```python
from build123d import *

# Parameters (mm, degrees)
SKETCH1_R               = 1.5
BOSS_EXTRUDE1_DEPTH     = 3.18
SKETCH1_6_R             = 1.5
BOSS_EXTRUDE2_DEPTH     = 1.59
CUT_EXTRUDE1_DEPTH      = 183.307082693
CUT_EXTRUDE1_DEPTH_BACK = 183.307082693
SKETCH2_R               = 1.725


with BuildPart() as part:
    # Sketch1 → Boss-Extrude1 (new body)
    with BuildSketch(Plane.XY):
        Polygon((46.2, 0), (0, 0), (0, -60), (46.2, -60), (46.2, -100), (106.2, -100), (106.2, -60), (152.4, -60), (152.4, 0), (106.2, 0), (106.2, 40), (46.2, 40), align=None)
        with Locations(Location((7.62, -55, 0), (0, 0, 180))):
            Circle(SKETCH1_R, mode=Mode.SUBTRACT)
        with Locations(Location((22.86, -55, 0), (0, 0, 180))):
            Circle(SKETCH1_R, mode=Mode.SUBTRACT)
        with Locations(Location((7.62, -45, 0), (0, 0, 180))):
            Circle(SKETCH1_R, mode=Mode.SUBTRACT)
        with Locations(Location((7.62, -35, 0), (0, 0, 180))):
            Circle(SKETCH1_R, mode=Mode.SUBTRACT)
        with Locations(Location((38.1, -55, 0), (0, 0, 180))):
            Circle(SKETCH1_R, mode=Mode.SUBTRACT)
        with Locations(Location((53.34, -55, 0), (0, 0, 180))):
            Circle(SKETCH1_R, mode=Mode.SUBTRACT)
        with Locations(Location((68.58, -55, 0), (0, 0, 180))):
            Circle(SKETCH1_R, mode=Mode.SUBTRACT)
        with Locations(Location((83.82, -55, 0), (0, 0, 180))):
            Circle(SKETCH1_R, mode=Mode.SUBTRACT)
        with Locations(Location((99.06, -55, 0), (0, 0, 180))):
            Circle(SKETCH1_R, mode=Mode.SUBTRACT)
        with Locations(Location((114.3, -55, 0), (0, 0, 180))):
            Circle(SKETCH1_R, mode=Mode.SUBTRACT)
        with Locations(Location((129.54, -55, 0), (0, 0, 180))):
            Circle(SKETCH1_R, mode=Mode.SUBTRACT)
        with Locations(Location((144.78, -55, 0), (0, 0, 180))):
            Circle(SKETCH1_R, mode=Mode.SUBTRACT)
        with Locations(Location((144.78, -45, 0), (0, 0, 180))):
            Circle(SKETCH1_R, mode=Mode.SUBTRACT)
        with Locations(Location((144.78, -35, 0), (0, 0, 180))):
            Circle(SKETCH1_R, mode=Mode.SUBTRACT)
        with Locations(Location((7.62, -25, 0), (0, 0, 180))):
            Circle(SKETCH1_R, mode=Mode.SUBTRACT)
        with Locations(Location((7.62, -15, 0), (0, 0, 180))):
            Circle(SKETCH1_R, mode=Mode.SUBTRACT)
        with Locations(Location((7.62, -5, 0), (0, 0, 180))):
            Circle(SKETCH1_R, mode=Mode.SUBTRACT)
        with Locations(Location((22.86, -5, 0), (0, 0, 180))):
            Circle(SKETCH1_R, mode=Mode.SUBTRACT)
        with Locations(Location((38.1, -5, 0), (0, 0, 180))):
            Circle(SKETCH1_R, mode=Mode.SUBTRACT)
        with Locations(Location((53.34, -5, 0), (0, 0, 180))):
            Circle(SKETCH1_R, mode=Mode.SUBTRACT)
        with Locations(Location((99.06, -5, 0), (0, 0, 180))):
            Circle(SKETCH1_R, mode=Mode.SUBTRACT)
        with Locations(Location((144.78, -25, 0), (0, 0, 180))):
            Circle(SKETCH1_R, mode=Mode.SUBTRACT)
        with Locations(Location((144.78, -15, 0), (0, 0, 180))):
            Circle(SKETCH1_R, mode=Mode.SUBTRACT)
        with Locations(Location((114.3, -5, 0), (0, 0, 180))):
            Circle(SKETCH1_R, mode=Mode.SUBTRACT)
        with Locations(Location((129.54, -5, 0), (0, 0, 180))):
            Circle(SKETCH1_R, mode=Mode.SUBTRACT)
        with Locations(Location((144.78, -5, 0), (0, 0, 180))):
            Circle(SKETCH1_R, mode=Mode.SUBTRACT)
        with Locations(Location((99.06, 35, 0), (0, 0, 180))):
            Circle(SKETCH1_R, mode=Mode.SUBTRACT)
        with Locations(Location((53.34, 8.333333333, 0), (0, 0, 180))):
            Circle(SKETCH1_R, mode=Mode.SUBTRACT)
        with Locations(Location((53.34, 21.666666667, 0), (0, 0, 180))):
            Circle(SKETCH1_R, mode=Mode.SUBTRACT)
        with Locations(Location((53.34, 35, 0), (0, 0, 180))):
            Circle(SKETCH1_R, mode=Mode.SUBTRACT)
        with Locations(Location((68.58, 35, 0), (0, 0, 180))):
            Circle(SKETCH1_R, mode=Mode.SUBTRACT)
        with Locations(Location((99.06, 8.333333333, 0), (0, 0, 180))):
            Circle(SKETCH1_R, mode=Mode.SUBTRACT)
        with Locations(Location((99.06, 21.666666667, 0), (0, 0, 180))):
            Circle(SKETCH1_R, mode=Mode.SUBTRACT)
        with Locations(Location((83.82, 35, 0), (0, 0, 180))):
            Circle(SKETCH1_R, mode=Mode.SUBTRACT)
        with Locations(Location((99.06, -68.333333333, 0), (0, 0, 180))):
            Circle(SKETCH1_R, mode=Mode.SUBTRACT)
        with Locations(Location((53.34, -95, 0), (0, 0, 180))):
            Circle(SKETCH1_R, mode=Mode.SUBTRACT)
        with Locations(Location((68.58, -95, 0), (0, 0, 180))):
            Circle(SKETCH1_R, mode=Mode.SUBTRACT)
        with Locations(Location((53.34, -81.666666667, 0), (0, 0, 180))):
            Circle(SKETCH1_R, mode=Mode.SUBTRACT)
        with Locations(Location((53.34, -68.333333333, 0), (0, 0, 180))):
            Circle(SKETCH1_R, mode=Mode.SUBTRACT)
        with Locations(Location((83.82, -95, 0), (0, 0, 180))):
            Circle(SKETCH1_R, mode=Mode.SUBTRACT)
        with Locations(Location((99.06, -95, 0), (0, 0, 180))):
            Circle(SKETCH1_R, mode=Mode.SUBTRACT)
        with Locations(Location((99.06, -81.666666667, 0), (0, 0, 180))):
            Circle(SKETCH1_R, mode=Mode.SUBTRACT)
    extrude(amount=BOSS_EXTRUDE1_DEPTH)

    # Sketch1_6 → Boss-Extrude2 (add)
    with BuildSketch(Plane.XY):
        with Locations(Location((7.62, -5, 0), (0, 0, 180))):
            Circle(SKETCH1_6_R)
        with Locations(Location((22.86, -5, 0), (0, 0, 180))):
            Circle(SKETCH1_6_R)
        with Locations(Location((7.62, -15, 0), (0, 0, 180))):
            Circle(SKETCH1_6_R)
        with Locations(Location((53.34, -5, 0), (0, 0, 180))):
            Circle(SKETCH1_6_R)
        with Locations(Location((38.1, -5, 0), (0, 0, 180))):
            Circle(SKETCH1_6_R)
        with Locations(Location((53.34, 8.333333333, 0), (0, 0, 180))):
            Circle(SKETCH1_6_R)
        with Locations(Location((53.34, 21.666666667, 0), (0, 0, 180))):
            Circle(SKETCH1_6_R)
        with Locations(Location((53.34, 35, 0), (0, 0, 180))):
            Circle(SKETCH1_6_R)
        with Locations(Location((68.58, 35, 0), (0, 0, 180))):
            Circle(SKETCH1_6_R)
        with Locations(Location((99.06, 35, 0), (0, 0, 180))):
            Circle(SKETCH1_6_R)
        with Locations(Location((83.82, 35, 0), (0, 0, 180))):
            Circle(SKETCH1_6_R)
        with Locations(Location((99.06, 8.333333333, 0), (0, 0, 180))):
            Circle(SKETCH1_6_R)
        with Locations(Location((99.06, 21.666666667, 0), (0, 0, 180))):
            Circle(SKETCH1_6_R)
        with Locations(Location((99.06, -5, 0), (0, 0, 180))):
            Circle(SKETCH1_6_R)
        with Locations(Location((114.3, -5, 0), (0, 0, 180))):
            Circle(SKETCH1_6_R)
        with Locations(Location((129.54, -5, 0), (0, 0, 180))):
            Circle(SKETCH1_6_R)
        with Locations(Location((144.78, -5, 0), (0, 0, 180))):
            Circle(SKETCH1_6_R)
        with Locations(Location((144.78, -15, 0), (0, 0, 180))):
            Circle(SKETCH1_6_R)
        with Locations(Location((144.78, -25, 0), (0, 0, 180))):
            Circle(SKETCH1_6_R)
        with Locations(Location((144.78, -35, 0), (0, 0, 180))):
            Circle(SKETCH1_6_R)
        with Locations(Location((144.78, -45, 0), (0, 0, 180))):
            Circle(SKETCH1_6_R)
        with Locations(Location((144.78, -55, 0), (0, 0, 180))):
            Circle(SKETCH1_6_R)
        with Locations(Location((129.54, -55, 0), (0, 0, 180))):
            Circle(SKETCH1_6_R)
        with Locations(Location((114.3, -55, 0), (0, 0, 180))):
            Circle(SKETCH1_6_R)
        with Locations(Location((99.06, -55, 0), (0, 0, 180))):
            Circle(SKETCH1_6_R)
        with Locations(Location((99.06, -68.333333333, 0), (0, 0, 180))):
            Circle(SKETCH1_6_R)
        with Locations(Location((99.06, -81.666666667, 0), (0, 0, 180))):
            Circle(SKETCH1_6_R)
        with Locations(Location((99.06, -95, 0), (0, 0, 180))):
            Circle(SKETCH1_6_R)
        with Locations(Location((83.82, -95, 0), (0, 0, 180))):
            Circle(SKETCH1_6_R)
        with Locations(Location((68.58, -95, 0), (0, 0, 180))):
            Circle(SKETCH1_6_R)
        with Locations(Location((53.34, -81.666666667, 0), (0, 0, 180))):
            Circle(SKETCH1_6_R)
        with Locations(Location((53.34, -95, 0), (0, 0, 180))):
            Circle(SKETCH1_6_R)
        with Locations(Location((53.34, -68.333333333, 0), (0, 0, 180))):
            Circle(SKETCH1_6_R)
        with Locations(Location((53.34, -55, 0), (0, 0, 180))):
            Circle(SKETCH1_6_R)
        with Locations(Location((38.1, -55, 0), (0, 0, 180))):
            Circle(SKETCH1_6_R)
        with Locations(Location((22.86, -55, 0), (0, 0, 180))):
            Circle(SKETCH1_6_R)
        with Locations(Location((7.62, -25, 0), (0, 0, 180))):
            Circle(SKETCH1_6_R)
        with Locations(Location((7.62, -35, 0), (0, 0, 180))):
            Circle(SKETCH1_6_R)
        with Locations(Location((7.62, -45, 0), (0, 0, 180))):
            Circle(SKETCH1_6_R)
        with Locations(Location((7.62, -55, 0), (0, 0, 180))):
            Circle(SKETCH1_6_R)
    extrude(amount=BOSS_EXTRUDE2_DEPTH)

    # Sketch2 → Cut-Extrude1 (cut, two sides: drawn at the far end of the back side and taken through both)
    with BuildSketch(Plane.XY.offset(3.18).offset(-CUT_EXTRUDE1_DEPTH_BACK)):
        with Locations((94.5382, -11.6618)):
            Circle(SKETCH2_R)
        with Locations((94.5382, -48.3382)):
            Circle(SKETCH2_R)
        with Locations((16.7, -30)):
            Circle(SKETCH2_R)
    extrude(amount=CUT_EXTRUDE1_DEPTH + CUT_EXTRUDE1_DEPTH_BACK, mode=Mode.SUBTRACT)


solid = part.part
```
Could you check a few things on this model? Use its own coordinates, in mm. A direction names the side the tool comes from. Round coordinates to 2 decimals unless told otherwise and drop trailing zeros. Write each loop counter-clockwise with the first axis right and the second up, starting at its lowest first coordinate (ties: lowest second). Pieces come first, ordered by that corner, then holes.
(1) Suppose I cut it at B-B on y = -30. Write out the boundary of the cut face in (x, z) (3 decimals), and give its area (3 significant figures).
Findings below:
outline: (0, 0) - (14.975, 0) - (14.975, 3.18) - (0, 3.18) - close; (18.425, 0) - (152.4, 0) - (152.4, 3.18) - (18.425, 3.18) - close
area: 474 mm2
(2) If I drill on probe 1 along Y at (x, z) = (84, 2.7); probe 2 along X at (y, z) = (-81, 1.8); probe 3 along X at (y, z) = (-55, 1.5), over which ranges is the centre line in solid material (lowest first)?
Findings below:
probe 1: y = -100 to -96.49, -93.51 to -56.49, -53.51 to 33.51, 36.49 to 40
probe 2: x = 46.2 to 52, 54.68 to 97.72, 100.4 to 106.2
probe 3: x = 0 to 67.08, 70.08 to 82.32, 85.32 to 152.4
(3) Suppose I cut it at C-C on z = 0.6. Write out the boundary of the cut face in (x, y) (3 decimals), and give its area (3 significant figures).
Findings below:
outline: (0, -60) - (46.2, -60) - (46.2, -100) - (106.2, -100) - (106.2, -60) - (152.4, -60) - (152.4, 0) - (106.2, 0) - (106.2, 40) - (46.2, 40) - (46.2, 0) - (0, 0) - close; hole circle Ø3.45 at (16.7, -30); hole circle Ø3 at (68.58, -55); hole circle Ø3 at (83.82, -55); hole circle Ø3.45 at (94.538, -48.338); hole circle Ø3.45 at (94.538, -11.662)
area: 13,900 mm2
(4) For pin 1 (2.5 mm diameter, centred on x = 144.78, y = -15, fed in from +Z), with a flat end and sliding along its axis, tell me the tip position at first contact or that it passes through.
Findings below:
pin 1: stops at z = 1.59
(5) Suppose I cut it at A-A on x = 16.7. Write out the boundary of the cut face in (y, z) (3 decimals), and give its area (3 significant figures).
Findings below:
outline: (-60, 0) - (-31.725, 0) - (-31.725, 3.18) - (-60, 3.18) - close; (-28.275, 0) - (0, 0) - (0, 3.18) - (-28.275, 3.18) - close
area: 180 mm2
(6) Which directions (+Z, -Z, +X, -X, +Y, -Y) give clear straight access to the entire face, cutting with the end or side of a thin tool? Please do faces 1 (the face through (130, 0, 2)), 2 (the face through (46.2, 20, 2)), 3 (the face through (129, -60, 2)), 4 (the face through (23, -60, 2)).
Findings below:
face 1: +Z, -Z, +X, +Y
face 2: +Z, -Z, -X, +Y
face 3: +Z, -Z, +X, -Y
face 4: +Z, -Z, -X, -Y
